For this review, take the finished solid that the model builds, in its own axes (mm). A direction names the side the tool comes from. Give positions to 0.01 mm unless a question says otherwise; leave off trailing zeros. Order: outer loops, then holes, each group sorted by start corner. A loop starts at its lowest first (then second) coordinate and runs counter-clockwise, first axis right, second up.
from build123d import *

# Parameters (mm, degrees)
SKETCH_W           = 150
SKETCH_H           = 200
PAD_DEPTH          = 50
SKETCH001_W        = 146
SKETCH001_H        = 196
PAD001_DEPTH       = 52
SKETCH002_W        = 142
SKETCH002_H        = 192
POCKET_DEPTH       = 50
SKETCH003_W        = 6
SKETCH003_H        = 6
POCKET001_DEPTH    = 5
SKETCH004_R        = 6
PAD002_DEPTH       = 50
POLARPATTERN_COUNT = 2


with BuildPart() as part:
    # Sketch → Pad (new body)
    with BuildSketch(Plane.XY):
        Rectangle(SKETCH_W, SKETCH_H)
    extrude(amount=PAD_DEPTH)

    # Sketch001 → Pad001 (join)
    with BuildSketch(Plane.XY):
        Rectangle(SKETCH001_W, SKETCH001_H)
    extrude(amount=PAD001_DEPTH)

    # Sketch002 → Pocket (cut)
    with BuildSketch(Plane.XY.offset(52)):
        Rectangle(SKETCH002_W, SKETCH002_H)
    extrude(amount=-POCKET_DEPTH, mode=Mode.SUBTRACT)

    # Sketch003 → Pocket001 (cut)
    with BuildSketch(Plane.XY):
        with Locations((52, 82)):
            Rectangle(SKETCH003_W, SKETCH003_H)
        with Locations((52, 64)):
            Rectangle(SKETCH003_W, SKETCH003_H)
        with Locations((52, 46)):
            Rectangle(SKETCH003_W, SKETCH003_H)
        with Locations((52, 28)):
            Rectangle(SKETCH003_W, SKETCH003_H)
        with Locations((-52, 82)):
            Rectangle(SKETCH003_W, SKETCH003_H)
        with Locations((-52, 64)):
            Rectangle(SKETCH003_W, SKETCH003_H)
        with Locations((-52, 46)):
            Rectangle(SKETCH003_W, SKETCH003_H)
        with Locations((-52, 28)):
            Rectangle(SKETCH003_W, SKETCH003_H)
    extrude(amount=POCKET001_DEPTH, mode=Mode.SUBTRACT)

    # Sketch004 → Pad002 (join)
    with BuildSketch(Plane.XY):
        with Locations((63, 88)):
            Circle(SKETCH004_R)
    pad002 = extrude(amount=PAD002_DEPTH)

    # Mirrored: Pad002 across Sketch004 V_Axis
    add(pad002.mirror(Plane(origin=(0, 0, 0), x_dir=(0, 0, 1), z_dir=(1, 0, 0))))

    # Mirrored001: Pad002 across Sketch004 H_Axis
    add(pad002.mirror(Plane.ZX))

    # PolarPattern: Pad002 ×2 about axis
    polarpattern_axis = Axis((0, 0, 0), (0, 0, 1))
    for i in range(1, POLARPATTERN_COUNT):
        add(pad002.rotate(polarpattern_axis, i * 360 / POLARPATTERN_COUNT))


solid = part.part
1) Draft analysis for pull direction X (two halves, no side actions). For faces 3 (the face through (-75, -1, 25)), 4 (the face through (75, -1, 25)), 5 (the face through (-1, 1, 2)), state which applies: +X half, -X half, draft (parallel to the pull), parting line (faces both ways), or undercut.
Answer sheet:
face 3: -X half
face 4: +X half
face 5: undercut
2) We need section D-D on x = 63. Give the boundary of the cut face in (y, z).
Answer sheet:
outline: (-100, 0) - (100, 0) - (100, 50) - (98, 50) - (98, 52) - (96, 52) - (96, 2) - (94, 2) - (94, 50) - (82, 50) - (82, 2) - (-82, 2) - (-82, 50) - (-94, 50) - (-94, 2) - (-96, 2) - (-96, 52) - (-98, 52) - (-98, 50) - (-100, 50) - close
3) We need section A-A on x = -52.5. Give the boundary of the cut face in (y, z).
Answer sheet:
outline: (-100, 0) - (25, 0) - (25, 2) - (-96, 2) - (-96, 52) - (-98, 52) - (-98, 50) - (-100, 50) - close; (31, 0) - (43, 0) - (43, 2) - (31, 2) - close; (49, 0) - (61, 0) - (61, 2) - (49, 2) - close; (67, 0) - (79, 0) - (79, 2) - (67, 2) - close; (85, 0) - (100, 0) - (100, 50) - (98, 50) - (98, 52) - (96, 52) - (96, 2) - (85, 2) - close
4) We need section B-B on y = 28.5. Give the boundary of the cut face in (x, z).
Answer sheet:
outline: (-75, 0) - (-55, 0) - (-55, 2) - (-71, 2) - (-71, 52) - (-73, 52) - (-73, 50) - (-75, 50) - close; (-49, 0) - (49, 0) - (49, 2) - (-49, 2) - close; (55, 0) - (75, 0) - (75, 50) - (73, 50) - (73, 52) - (71, 52) - (71, 2) - (55, 2) - close
5) Clearance check with flat-ended pins moving along their axes: pin 1 (0.6 mm diameter, centred on y = -21.5, z = 51, fed in from -X); pin 2 (0.6 mm diameter, centred on x = 23, z = 50.5, fed in from -Y); pin 3 (1 mm diameter, centred on y = 42.5, z = 51, fed in from +X). State where each tip first meets the part, or that it passes through.
Answer sheet:
pin 1: stops at x = -73
pin 2: stops at y = -98
pin 3: stops at x = 73
6) We need section C-C on z = 11.5. Give the boundary of the cut face in (x, y).
Answer sheet:
outline: (-75, -100) - (75, -100) - (75, 100) - (-75, 100) - close; circle Ø12 at (-63, -88); circle Ø12 at (-63, 88); circle Ø12 at (63, -88); circle Ø12 at (63, 88); hole (-71, -96) - (71, -96) - (71, 96) - (-71, 96) - close
7) Tool access review of faces 1 (the face through (1, -1, 0)), 2 (the face through (58.58, 92.06, 25.66)): name each direction out of +Z, -Z, +X, -X, +Y, -Y from which nothing blocks a thin tool from reaching the whole face with its end or side.
Answer sheet:
face 1: -Z, +X, -X, +Y, -Y
face 2: +Z
8) To check wall thickness, follow line 1 (X direction, y = 42, z = 33); line 2 (Y direction, x = 22, z = 36.5); line 3 (Z direction, x = 16, y = -42.5). State the ranges of each line that lie inside material, in increasing order.
Answer sheet:
line 1: x = -75 to -71, 71 to 75
line 2: y = -100 to -96, 96 to 100
line 3: z = 0 to 2
